For this review, take the finished solid that the model builds, in its own axes (mm). A direction names the side the tool comes from. Round coordinates to 2 decimals unless told otherwise and drop trailing zeros. Loops run counter-clockwise (first coordinate to the right, second up) from the corner with the lowest first, then second, coordinate; pieces in that order, holes last. Notation, with made-up numbers: (-23, 23.25) -> (-18, 23.25) arc R30 cw to (-18, 49.25) -> close; hole circle Ø1 at (30, -26.5). An arc over 180 degrees is marked (long way). One line per question, with ' | ' between items. Start each with the question number.
1. Consider section D-D (z = 13.25). Write out the cut boundary in (x, y).
2. Draft analysis for pull direction X (two halves, no side actions). For faces 4 (the face through (3.755, 7.93, 11.923)), 5 (the face through (-6, 2, 1)), 6 (the face through (11.2, 13, -2.8)), state which applies: pulls with the +X half, pulls with the -X half, needs draft (parallel to the pull), parting line crosses it, or undercut.
3. Consider section C-C (y = 7.75). Write out the cut boundary in (x, z).
4. Consider section B-B (x = 0). Write out the cut boundary in (y, z).
5. Wall thickness on line 1 along X through (y, z) = (7.75, 0); line 2 along Y through (x, z) = (-10.25, -7.75); line 3 along Z through (x, y) = (-4.75, 5): over which ranges is each line inside the solid? List them lowest first.
6. For faces 1 (the face through (6, 2, -1)), 2 (the face through (-2, 3, 2)), 3 (the face through (-3, 0, 3)), list the 3-axis set-ups (+Z, -Z, +X, -X, +Y, -Y) from which the entire face can be reached by the end or side of a thin tool; tool diameter is ignored.
7. Consider section A-A (z = 0). Write out the cut boundary in (x, y), and give its area (3 significant figures).
8. For pin 1 Ø13.5 at (x, z) = (0, 0) entering from +Y; pin 2 Ø3.5 at (y, z) = (1, 6) entering from -X; pin 3 Ø2.5 at (x, y) = (-6, 2) entering from -Z, all flat-tipped, find the tip position at first contact; note any pin that passes through.
```python
from build123d import *

# Parameters (mm, degrees)
SKETCH1_R           = 14.7
BOSS_EXTRUDE1_DEPTH = 3
SKETCH3_W           = 21.4
SKETCH3_H           = 2
CUT_EXTRUDE1_DEPTH  = 3
SKETCH4_W           = 2
SKETCH4_H           = 21.4
CUT_EXTRUDE2_DEPTH  = 3
SKETCH5_R           = 12.5
BOSS_EXTRUDE3_DEPTH = 10
SKETCH6_R           = 11.27
CUT_EXTRUDE3_DEPTH  = 10


with BuildPart() as part:
    # Sketch1 → Boss-Extrude1 (new body)
    with BuildSketch(Plane(origin=(0, 0, 0), x_dir=(1, 0, 0), z_dir=(0, 1, 0))):
        with Locations(Location((0, 0, 0), (0, 0, 270))):
            Circle(SKETCH1_R)
    extrude(amount=BOSS_EXTRUDE1_DEPTH)

    # Sketch3 → Cut-Extrude1 (cut)
    with BuildSketch(Plane(origin=(0, 3, 0), x_dir=(1, 0, 0), z_dir=(0, 1, 0))):
        Rectangle(SKETCH3_W, SKETCH3_H)
    extrude(amount=-CUT_EXTRUDE1_DEPTH, mode=Mode.SUBTRACT)

    # Sketch4 → Cut-Extrude2 (cut)
    with BuildSketch(Plane(origin=(0, 3, 0), x_dir=(1, 0, 0), z_dir=(0, 1, 0))):
        Rectangle(SKETCH4_W, SKETCH4_H)
    extrude(amount=-CUT_EXTRUDE2_DEPTH, mode=Mode.SUBTRACT)

    # Sketch5 → Boss-Extrude3 (add)
    with BuildSketch(Plane(origin=(0, 3, 0), x_dir=(1, 0, 0), z_dir=(0, 1, 0))):
        with Locations(Location((0, 0, 0), (0, 0, 270))):
            Circle(SKETCH5_R)
    extrude(amount=BOSS_EXTRUDE3_DEPTH)

    # Sketch6 → Cut-Extrude3 (cut)
    with BuildSketch(Plane(origin=(0, 13, 0), x_dir=(1, 0, 0), z_dir=(0, 1, 0))):
        with Locations(Location((0, 0, 0), (0, 0, 270))):
            Circle(SKETCH6_R)
    extrude(amount=-CUT_EXTRUDE3_DEPTH, mode=Mode.SUBTRACT)


solid = part.part
```
Answer block:
1) outline: (-6.37, 0) -> (6.37, 0) -> (6.37, 3) -> (-6.37, 3) -> close
2) face 4: parting line crosses it | face 5: undercut | face 6: needs draft
3) outline: circle Ø25 at (0, 0); hole circle Ø22.54 at (0, 0)
4) outline: (0, -14.7) -> (3, -14.7) -> (3, -12.5) -> (13, -12.5) -> (13, -11.27) -> (3, -11.27) -> (3, -10.7) -> (0, -10.7) -> close; (0, 10.7) -> (3, 10.7) -> (3, 11.27) -> (13, 11.27) -> (13, 12.5) -> (3, 12.5) -> (3, 14.7) -> (0, 14.7) -> close
5) line 1: x = -12.5 to -11.27, 11.27 to 12.5 | line 2: y = 0 to 3 | line 3: z = -11.56 to -10.22, 10.22 to 11.56
6) face 1: +Y, -Y | face 2: +Y | face 3: +Z, -Z, +X, -X, -Y
7) outline: (-14.7, 0) -> (-10.7, 0) -> (-10.7, 3) -> (-11.27, 3) -> (-11.27, 13) -> (-12.5, 13) -> (-12.5, 3) -> (-14.7, 3) -> close; (10.7, 0) -> (14.7, 0) -> (14.7, 3) -> (12.5, 3) -> (12.5, 13) -> (11.27, 13) -> (11.27, 3) -> (10.7, 3) -> close | area: 48.6 mm2
8) pin 1: stops at y = 3 | pin 2: stops at x = -14.07 | pin 3: stops at z = -13.91
